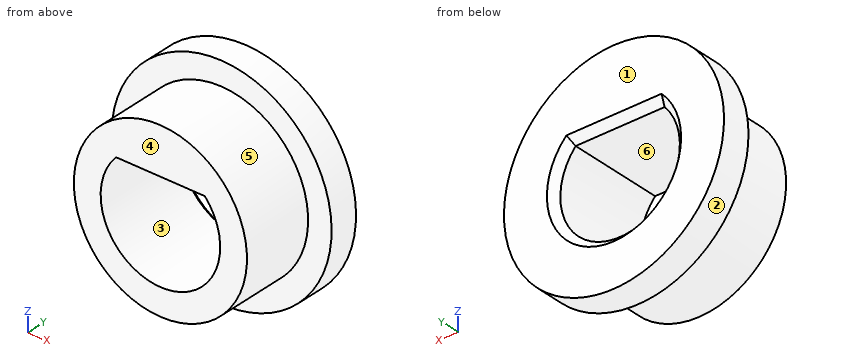
from build123d import *

# Parameters (mm, degrees)
SCHNITT_LINEAR_AUSTRAGEN1_DEPTH = 13.708265027
FASE1_SIZE                      = 0.5


with BuildPart() as part:
    # Skizze1 → Rotation1 (revolve)
    with BuildSketch(Plane.XY, mode=Mode.PRIVATE) as rotation1_sk:
        Polygon((0, 0), (5.9, 0), (5.9, 5), (7.5, 5), (7.5, 7), (0, 7), align=None)
    revolve(rotation1_sk.sketch.rotate(Axis((0, 0, 0), (0, -1, 0)), 90), axis=Axis((0, 0, 0), (0, -1, 0)))

    # Skizze2 → Schnitt-Linear austragen1 (cut, through all)
    with BuildSketch(Plane(origin=(0, 7, 0), x_dir=(1, 0, 0), z_dir=(0, 1, 0))):
        with BuildLine():
            Line((-3.029851482, -2.725), (3.029851482, -2.725))
            ThreePointArc((3.029851482, -2.725), (0, 4.075), (-3.029851482, -2.725))
        make_face()
    extrude(amount=-SCHNITT_LINEAR_AUSTRAGEN1_DEPTH, mode=Mode.SUBTRACT)

    # Fase1
    fase1_edges = [part.edges().sort_by_distance(p)[0] for p in [
        (0, 7, -4.075),
        (0, 7, 2.725),
    ]]
    chamfer(fase1_edges, length=FASE1_SIZE)


solid = part.part
Source: CAD feature listing. Evaluate the final solid. Frame: model axes, mm. Face numbers are marked on the shaded views. A direction names the side the tool comes from. Give positions to 0.01 mm unless a question says otherwise; leave off trailing zeros. Write each loop counter-clockwise with the first axis right and the second up, starting at its lowest first coordinate (ties: lowest second). Pieces come first, ordered by that corner, then holes. Notation, with made-up numbers: M 65.25,-30.5 L 115.25,-30.5 A15 cw 115.25,-20.5 Z; hole C 77,54 d2. An arc over 180 degrees is marked long. Return JSON: item names as keys, results as strings. Group by question number.
1) Ray query, L1, parallel to X at y = 5.25, z = 0 (3 decimals); L2, parallel to X at y = 2.25, z = 0 (3 decimals); L3, parallel to Y at x = -0.75, z = 7.25. Return the intervals inside material, ascending.
2) Cut plane B-B, the plane z = 0. Output: boundary loops of the cut face in (x, y) (3 decimals), then the cut area to 3 significant figures.
3) First-contact query: pin 1 Ø1.5 at (x, y) = (-3, 1) entering from +Z; pin 2 Ø1.8 at (x, y) = (1.5, 4.5) entering from -Z. Flat tips, straight axial feed; report the tip coordinate or a pass-through.
4) Cut plane D-D, the plane z = 4.5. Output: boundary loops of the cut face in (x, y), then the cut area to 3 significant figures.
5) Cut plane A-A, the plane x = 0. Output: boundary loops of the cut face in (y, z) (3 decimals).
6) Cut plane C-C, the plane y = 3. Output: boundary loops of the cut face in (x, z) (3 decimals).
7) Draft query along Z for the marked faces 1, 2 and 3. Return one class per face: released by +Z, released by -Z, zero draft, split by the parting line, or undercut.
8) Set-up query: the marked faces 4, 5 and 6. Return all of +Z, -Z, +X, -X, +Y, -Y with unobstructed straight access to the full face (end or side cutting, diameter ignored); none if empty.
Data:
{
 "1": {"L1": "x = -7.5 to -4.075, 4.075 to 7.5", "L2": "x = -5.9 to -4.075, 4.075 to 5.9", "L3": "y = 5 to 7"},
 "2": {"outline": "M -7.5,5 L -5.9,5 L -5.9,0 L -4.075,0 L -4.075,6.5 L -4.575,7 L -7.5,7 Z; M 4.075,0 L 5.9,0 L 5.9,5 L 7.5,5 L 7.5,7 L 4.575,7 L 4.075,6.5 Z", "area": "31.7 mm²"},
 "3": {"pin 1": "stops at z = 5.45", "pin 2": "stops at z = -7.46"},
 "4": {"outline": "M -6,5 L -3.82,5 L -3.82,0 L 3.82,0 L 3.82,5 L 6,5 L 6,7 L -6,7 Z", "area": "62.2 mm²"},
 "5": {"outline": "M 0,-5.9 L 5,-5.9 L 5,-7.5 L 7,-7.5 L 7,-4.575 L 6.5,-4.075 L 0,-4.075 Z; M 0,2.725 L 6.5,2.725 L 7,3.225 L 7,7.5 L 5,7.5 L 5,5.9 L 0,5.9 Z"},
 "6": {"outline": "C 0,0 d11.8; hole M -3.03,2.725 A4.075 ccw long 3.03,2.725 Z"},
 "7": {"face 1": "zero draft", "face 2": "split by the parting line", "face 3": "undercut"},
 "8": {"face 4": "+Z, -Z, +X, -X, -Y", "face 5": "-Y", "face 6": "+Y, -Y"}
}
